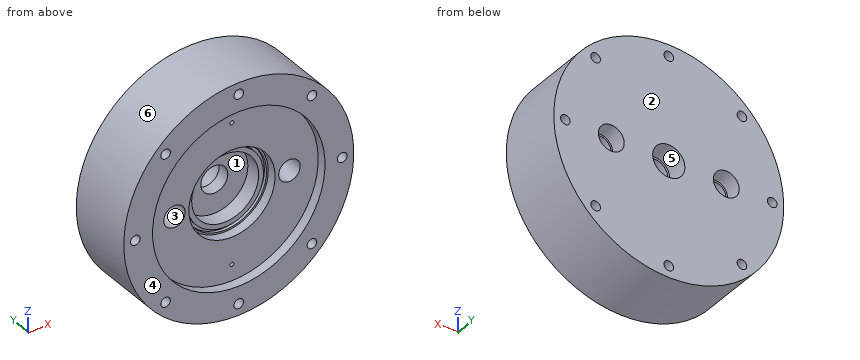
```python
from build123d import *

# Parameters (mm, degrees)
F_3_8_NPT_TAPPED_HOLE1_AT_2_COUNT = 2
F_3_8_NPT_TAPPED_HOLE1_AT_2_PITCH = 76.2
BOLT_HOLES_PROFILE_R              = 3.175
BOLT_HOLES_DEPTH                  = 117.570504417
DOWEL_HOLES_PROFILE_R             = 1.27
DOWEL_HOLES_DEPTH                 = 2.54


with BuildPart() as part:
    # Main Shape Profile → Main Shape (revolve)
    with BuildSketch(Plane.XY, mode=Mode.PRIVATE) as main_shape_sk:
        Polygon((0, 44.45), (0, 22.86), (22.225, 22.86), (22.225, 12.7), (25.4, 12.7), (25.4, 14.732), (27.432, 14.732), (27.432, 12.7), (28.575, 12.7), (28.575, 6.35), (57.15, 6.35), (57.15, 0), (76.2, 0), (76.2, 44.45), align=None)
    revolve(main_shape_sk.sketch.rotate(Axis((0, 0, 0), (0, -1, 0)), 90), axis=Axis((0, 0, 0), (0, -1, 0)))

    # Sketch3 → 1/2 NPT Tapped Hole1 (revolve, cut)
    with BuildSketch(Plane(origin=(0, 44.45, 0), x_dir=(0, 0, 1), z_dir=(1, 0, 0))):
        Polygon((0, 0), (0, 44.45), (8.9281, 44.45), (8.9281, 13.462), (10.261665792, 13.462), (10.6647361, 0), align=None)
    revolve(axis=Axis((0, 50.8, 0), (0, -1, 0)), mode=Mode.SUBTRACT)

    # Sketch4 → 3/8 NPT Tapped Hole1 (revolve, cut)
    with BuildSketch(Plane(origin=(-38.1, 44.45, 0), x_dir=(0, 0, 1), z_dir=(1, 0, 0))):
        Polygon((0, 0), (0, 44.45), (7.1374, 44.45), (7.1374, 10.414), (8.263205494, 10.414), (8.5750146, 0), align=None)
    f_3_8_npt_tapped_hole1 = revolve(axis=Axis((-38.1, 50.8, 0), (0, -1, 0)), mode=Mode.SUBTRACT)

    # 3/8 NPT Tapped Hole1 at 2: 3/8 NPT Tapped Hole1 ×2
    with Locations(*[(i * F_3_8_NPT_TAPPED_HOLE1_AT_2_PITCH, 0, 0) for i in range(1, F_3_8_NPT_TAPPED_HOLE1_AT_2_COUNT)]):
        add(f_3_8_npt_tapped_hole1, mode=Mode.SUBTRACT)

    # Bolt Holes Profile → Bolt Holes (cut, through all)
    with BuildSketch(Plane(origin=(0, 44.45, 0), x_dir=(1, 0, 0), z_dir=(0, 1, 0))):
        with Locations(Location((0, 68.58, 0), (0, 0, 270))):
            Circle(BOLT_HOLES_PROFILE_R)
        with Locations(Location((48.493383054, 48.493383054, 0), (0, 0, 270))):
            Circle(BOLT_HOLES_PROFILE_R)
        with Locations(Location((68.58, 0, 0), (0, 0, 270))):
            Circle(BOLT_HOLES_PROFILE_R)
        with Locations(Location((48.493383054, -48.493383054, 0), (0, 0, 270))):
            Circle(BOLT_HOLES_PROFILE_R)
        with Locations(Location((0, -68.58, 0), (0, 0, 270))):
            Circle(BOLT_HOLES_PROFILE_R)
        with Locations(Location((-48.493383054, -48.493383054, 0), (0, 0, 270))):
            Circle(BOLT_HOLES_PROFILE_R)
        with Locations(Location((-68.58, 0, 0), (0, 0, 270))):
            Circle(BOLT_HOLES_PROFILE_R)
        with Locations(Location((-48.493383054, 48.493383054, 0), (0, 0, 270))):
            Circle(BOLT_HOLES_PROFILE_R)
    extrude(amount=-BOLT_HOLES_DEPTH, mode=Mode.SUBTRACT)

    # Dowel Holes Profile → Dowel Holes (cut)
    with BuildSketch(Plane.XZ.offset(-6.35)):
        with Locations(Location((0, 46.355, 0), (0, 0, 270))):
            Circle(DOWEL_HOLES_PROFILE_R)
        with Locations(Location((0, -46.355, 0), (0, 0, 270))):
            Circle(DOWEL_HOLES_PROFILE_R)
    extrude(amount=-DOWEL_HOLES_DEPTH, mode=Mode.SUBTRACT)


solid = part.part
```
The model under review builds one solid part; all positions refer to its coordinate system, in mm. Face numbers are marked on the shaded views. A direction names the side the tool comes from. Round coordinates to 2 decimals unless told otherwise and drop trailing zeros. Write each loop counter-clockwise with the first axis right and the second up, starting at its lowest first coordinate (ties: lowest second). Pieces come first, ordered by that corner, then holes.
(1) We need section C-C on z = 68.58. Give the boundary of the cut face in (x, y) (3 decimals).
(2) We need section B-B on y = 39.5. Give the number of separate pieces and of enclosed holes in the cut face, and give its area (3 significant figures).
(3) Machinability: for the marked faces 1 and 2, which of the approach directions +Z, -Z, +X, -X, +Y, -Y give a long, thin tool a straight path to every point of the face, cutting with its end or side? Answer none if there is none.
(4) Wall thickness on L1, parallel to X at y = 25, z = 0 (3 decimals); L2, parallel to Z at x = 49, y = 4; L3, parallel to Y at x = 17, z = 30.5: over which ranges is each line inside the solid? List them lowest first.
(5) We need section D-D on z = -37.5. Give the boundary of the cut face in (x, y).
(6) Insertion check: pin 1 (4 mm diameter, centred on y = 20.5, z = 57, fed in from -X); pin 2 (5 mm diameter, centred on x = 68.58, z = 0, fed in from +Y); pin 3 (13.5 mm diameter, centred on x = -6.5, z = 4.5, fed in from -Y); pin 4 (1 mm diameter, centred on x = -27.5, y = 12.5, fed in from +Z). Each pin has a flat end and moves straight along its axis. Give the tip position at first contact, or say it passes through.
(7) We need section A-A on x = 68.58. Give the boundary of the cut face in (y, z) (3 decimals).
(8) Mouldability with a two-part tool opening along Z and no side actions: class the marked faces 3, 4, 5 and 6 as +Z half, -Z half, draft (parallel to the pull), parting line (faces both ways), or undercut.
Findings below:
1. outline: (-33.215, 0) - (-3.175, 0) - (-3.175, 44.45) - (-33.215, 44.45) - close; (3.175, 0) - (33.215, 0) - (33.215, 44.45) - (3.175, 44.45) - close
2. separate pieces: 1
2. enclosed holes: 11
2. area: 17,200 mm2
3. face 1: -Y
3. face 2: +Z, -Z, +X, -X, +Y
4. L1: x = -76.2 to -71.755, -65.405 to -45.237, -30.963 to -8.928, 8.928 to 30.963, 45.237 to 65.405, 71.755 to 76.2
4. L2: z = -58.36 to -51.63, -45.36 to -29.41, 29.41 to 45.36, 51.63 to 58.36
4. L3: y = 6.35 to 44.45
5. outline: (-66.33, 0) - (-43.13, 0) - (-43.13, 6.35) - (43.13, 6.35) - (43.13, 0) - (66.33, 0) - (66.33, 44.45) - (-66.33, 44.45) - close
6. pin 1: stops at x = -52.74
6. pin 2: passes through
6. pin 3: stops at y = 22.86
6. pin 4: stops at z = 71.26
7. outline: (0, -33.215) - (44.45, -33.215) - (44.45, -3.175) - (0, -3.175) - close; (0, 3.175) - (44.45, 3.175) - (44.45, 33.215) - (0, 33.215) - close
8. face 3: undercut
8. face 4: draft
8. face 5: undercut
8. face 6: parting line
